Read the model definition and answer for the solid it produces. Units are mm, in the model's axes. A direction names the side the tool comes from. Coordinates: 2 decimals unless noted, no trailing zeros. Write each loop counter-clockwise with the first axis right and the second up, starting at its lowest first coordinate (ties: lowest second). Pieces come first, ordered by that corner, then holes.
(1) Given pin 1 (6 mm diameter, centred on y = 54, z = 80.8, fed in from -X); pin 2 (8 mm diameter, centred on y = 53.5, z = 82.5, fed in from +X); pin 3 (3.5 mm diameter, centred on y = 4.5, z = 4, fed in from +X), each flat-ended and moving along its own axis, determine where each tip first touches the part or whether it passes through.
(2) The mould has two halves that part along Z. Classify faces 4 (the cylindrical face through (0.2, 68.5, 40.9)), 5 (the cylindrical face through (0.25, 62.46, 1.15)), 6 (the flat face through (11.65, 3, 4)): +Z half, -Z half, draft (parallel to the pull), parting line (faces both ways), or undercut.
(3) Find the intervals of material crossed by probe 1 along Z at (x, y) = (-1, 54); probe 2 along Z at (x, y) = (-15, 5); probe 3 along Z at (x, y) = (13.5, 49.5), in increasing order.
(4) Which of the six approach directions +Z, -Z, +X, -X, +Y, -Y give full straight-line access (tool end or side, diameter ignored) to faces 1 (the flat face through (-11.65, 3, 4)), 2 (the flat face through (17.65, 35, 42)), 3 (the cylindrical face through (14.69, 57.57, 81.27))?
(5) Section B-B on z = 54 is taken. Write down the section's boundary in (x, y), then the cut area to 3 significant figures.
(6) Section A-A on z = -44 is taken. Write down the section's boundary in (x, y).
from build123d import *

# Parameters (mm, degrees)
ESQUISSE2_R      = 2.25
EXTRUSION1_DEPTH = 17.65
ESQUISSE3_R      = 3.6
EXTRUSION2_DEPTH = 6
ESQUISSE4_R      = 3.5
EXTRUSION3_DEPTH = 55
ESQUISSE6_R      = 3.5
EXTRUSION4_DEPTH = 150


with BuildPart() as part:
    # Esquisse2 → Extrusion1 (new, symmetric)
    with BuildSketch(Plane(origin=(0, 0, 0), x_dir=(0, 0, -1), z_dir=(1, 0, 0))):
        with BuildLine():
            Line((-67.523044738, 1.523044738), (-84.476955262, 18.476955262))
            ThreePointArc((-84.476955262, 18.476955262), (-85.604173569, 20.163956676), (-86, 22.153910524))
            Line((-86, 22.153910524), (-86, 54))
            ThreePointArc((-86, 54), (-84.476955262, 57.676955262), (-80.8, 59.2))
            ThreePointArc((-80.8, 59.2), (-79.677669391, 62.426857966), (-76.795149102, 64.260792292))
            ThreePointArc((-76.795149102, 64.260792292), (-40.4, 68.5), (-4.004850898, 64.260792292))
            ThreePointArc((-4.004850898, 64.260792292), (-1.122330609, 62.426857966), (0, 59.2))
            Line((0, 59.2), (0, 5.2))
            ThreePointArc((0, 5.2), (-1.523044738, 1.523044738), (-5.2, 0))
            Line((-5.2, 0), (-63.846089476, 0))
            ThreePointArc((-63.846089476, 0), (-65.836043324, 0.395826431), (-67.523044738, 1.523044738))
        make_face()
        with Locations((-80.8, 54)):
            Circle(ESQUISSE2_R, mode=Mode.SUBTRACT)
        with Locations((-5.2, 5.2)):
            Circle(ESQUISSE2_R, mode=Mode.SUBTRACT)
    extrude(amount=EXTRUSION1_DEPTH, both=True)

    # Esquisse3 → Extrusion2 (cut)
    with BuildSketch(Plane(origin=(17.65, 0, 0), x_dir=(0, 0, -1), z_dir=(1, 0, 0))):
        with Locations((-80.8, 54)):
            Circle(ESQUISSE3_R)
        with Locations((-5.2, 5.2)):
            Circle(ESQUISSE3_R)
    extrusion2 = extrude(amount=-EXTRUSION2_DEPTH, mode=Mode.SUBTRACT)

    # Symétrie1: Extrusion2 across plane
    add(extrusion2.mirror(Plane(origin=(0, 0, 0), x_dir=(0, 0, 1), z_dir=(1, 0, 0))), mode=Mode.SUBTRACT)

    # Esquisse4 → Extrusion3 (add)
    with BuildSketch(Plane(origin=(0, 0, 0), x_dir=(-1, 0, 0), z_dir=(0, 0, -1))):
        with Locations(Location((0, 29.5, 0), (0, 0, 270))):
            Circle(ESQUISSE4_R)
    extrude(amount=EXTRUSION3_DEPTH)

    # Esquisse6 → Extrusion4 (add)
    with BuildSketch(Plane(origin=(-8.7708228, 2.891030086, 0), x_dir=(0, 0, -1), z_dir=(0.9497362687231024, -0.3130511457764037, 0))):
        with Locations(Location((50.51548438, 28.017219927, 0), (0, 0, 90))):
            Circle(ESQUISSE6_R)
    extrude(amount=EXTRUSION4_DEPTH)


solid = part.part
Response:
1. pin 1: stops at x = -11.65
1. pin 2: stops at x = 17.65
1. pin 3: stops at x = 11.65
2. face 4: parting line
2. face 5: -Z half
2. face 6: undercut
3. probe 1: z = 0 to 78.55, 83.05 to 86
3. probe 2: z = 0 to 1.61, 8.79 to 71
3. probe 3: z = 0 to 86
4. face 1: -X
4. face 2: +Z, +X, +Y, -Y
4. face 3: +X
5. outline: (-17.65, 0) - (17.65, 0) - (17.65, 67.91) - (-17.65, 67.91) - close
5. area: 2,400 mm2
6. outline: circle Ø7 at (0, 29.5)
